For this review, take the finished solid that the model builds, in its own axes (mm). Face numbers are marked on the shaded views. A direction names the side the tool comes from. Give positions to 0.01 mm unless a question says otherwise; leave off trailing zeros. Order: outer loops, then holes, each group sorted by start corner. A loop starts at its lowest first (then second) coordinate and runs counter-clockwise, first axis right, second up.
Autodesk Inventor part; units mm, degrees
ref_plane "YZ Plane" through (0, 0, 0) normal (1, 0, 0) x (0, 1, 0)
ref_plane "XZ Plane" through (0, 0, 0) normal (0, 1, 0) x (-1, 0, 0)
ref_plane "XY Plane" through (0, 0, 0) normal (0, 0, 1) x (1, 0, 0)
sketch "スケッチ3" plane through (0, 0, 0) normal (0, 1, 0) x (-1, 0, 0)
  circle A0 centre (0, 0) radius 3.85
  line L0 (11, -4) -> (4.4721, -4)
  line L1 (-11, -4) -> (-11, -6)
  line L2 (-11, -6) -> (11, -6)
  line L3 (11, -6) -> (11, -4)
  arc A1 (4.4721, -4) -> (-4.4721, -4) centre (0, 0) ccw
  line L4 (-4.4721, -4) -> (-11, -4)
  point P0 (0, -4)
  point P1 (0, -6)
  dimension "d12" = 7.7
  dimension "d14" = 22
  dimension "d15" = 2
  dimension "d16" = 6
extrude "押し出し3" add sketch "スケッチ3" along normal blind 10
sketch "スケッチ4" plane through (4.4721, 0, -4) normal (0, 0, 1) x (1, 0, 0)
  circle A0 centre (4.0279, 7.5) radius 1.05
  circle A1 centre (-12.9721, 2.5) radius 1.05
  line L0 (-15.4721, 0) -> (-15.4721, 10)
  line L1 (6.5279, 0) -> (6.5279, 10)
  line L2 (0, 10) -> (6.5279, 10)
  line L3 (-15.4721, 0) -> (-8.9443, 0)
  line L4 (0, 0) -> (0, 10)
  line L5 (0, 0) -> (6.5279, 0)
  line L6 (0, 0) -> (6.5279, 0)
  line L7 (6.5279, 0) -> (6.5279, 10)
  line L8 (0, 10) -> (6.5279, 10)
  line L9 (0, 0) -> (0, 10)
  line L10 (6.5279, 5) -> (0, 5)
  line L11 (0, 0) -> (6.5279, 0)
  line L12 (6.5279, 5) -> (6.5279, 0)
  line L13 (6.5279, 0) -> (0, 0)
  line L14 (1.5279, 0) -> (-10.4721, 0)
  line L15 (0, 0) -> (0, 5)
  line L16 (-15.4721, 0) -> (-8.9443, 0)
  line L17 (-8.9443, 0) -> (-8.9443, 10)
  line L18 (-15.4721, 10) -> (-8.9443, 10)
  line L19 (-15.4721, 0) -> (-15.4721, 10)
  line L20 (-15.4721, 0) -> (-15.4721, 10)
  line L21 (-15.4721, 10) -> (-8.9443, 10)
  line L22 (-15.4721, 5) -> (-8.9443, 5)
  line L23 (-8.9443, 5) -> (-8.9443, 10)
  line L24 (-8.9443, 10) -> (-15.4721, 10)
  line L25 (-15.4721, 10) -> (-15.4721, 5)
  point P0 (-4.4721, 0)
  dimension "d19" = 2.1
  dimension "d20" = 2.1
  dimension "d21" = 2.5
  dimension "d22" = 2.5
  dimension "d29" = 2.5
  dimension "d30" = 2.5
  dimension "d35" = 17
extrude "押し出し4" cut sketch "スケッチ4" against normal blind 10 contours A0 | A1
sketch "スケッチ5" plane through (0, 10, 0) normal (0, 1, 0) x (1, 0, 0)
  line L0 (-1.5, 0) -> (1.5, 0)
  line L1 (1.5, 0) -> (1.5, 10)
  line L2 (1.5, 10) -> (-1.5, 10)
  line L3 (-1.5, 10) -> (-1.5, 0)
  point P0 (0, 0)
  point P1 (0, 0)
  dimension "d25" = 3
  dimension "d26" = 10
extrude "押し出し5" cut sketch "スケッチ5" against normal blind 10
extrude "押し出し6" cut sketch "スケッチ4" against normal blind 2 contours L4 L10 L1 L5
extrude "押し出し7" cut sketch "スケッチ4" against normal blind 2 contours L0 L18 L17 L22
properties part number "Ω型"
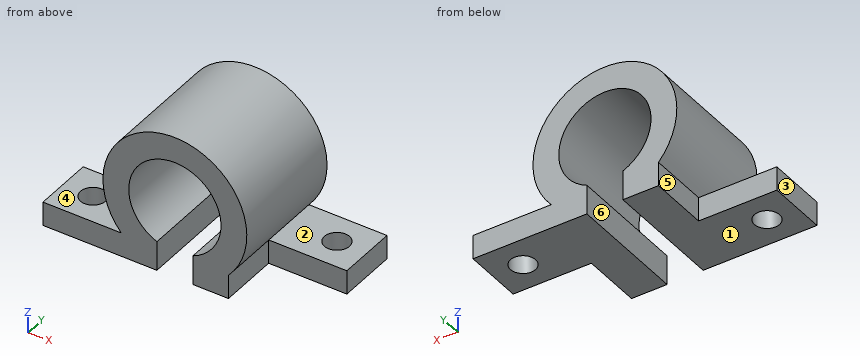
1) Tool access review of the marked faces 4, 5 and 6: name each direction out of +Z, -Z, +X, -X, +Y, -Y from which nothing blocks a thin tool from reaching the whole face with its end or side.
Answer sheet:
face 4: -X, +Y, -Y
face 5: -Z, -X, +Y
face 6: -Z, +Y, -Y
2) We need section A-A on x = 8.5. Give the boundary of the cut face in (y, z).
Answer sheet:
outline: (5, -6) - (6.45, -6) - (6.45, -4) - (5, -4) - close; (8.55, -6) - (10, -6) - (10, -4) - (8.55, -4) - close
3) We need section D-D on y = 4.75. Give the boundary of the cut face in (x, z).
Answer sheet:
outline: (-11, -6) - (-1.5, -6) - (-1.5, -3.55) arc R3.85 cw (long way) to (1.5, -3.55) - (1.5, -6) - (4.47, -6) - (4.47, -4) arc R6 ccw (long way) to (-4.47, -4) - (-11, -4) - close
4) Draft analysis for pull direction Z (two halves, no side actions). For the marked faces 1, 2 and 3, state which applies: +Z half, -Z half, draft (parallel to the pull), parting line (faces both ways), or undercut.
Answer sheet:
face 1: -Z half
face 2: undercut
face 3: draft
5) Clearance check with flat-ended pins moving along their axes: pin 1 (1.5 mm diameter, centred on x = 7.5, y = 8, fed in from +Z); pin 2 (1.2 mm diameter, centred on y = 3.5, z = -5, fed in from +X); pin 3 (1.5 mm diameter, centred on x = 5, y = 5.5, fed in from +Z). State where each tip first meets the part, or that it passes through.
Answer sheet:
pin 1: stops at z = -4
pin 2: stops at x = 4.47
pin 3: stops at z = 4.24
6) We need section C-C on z = -1.5. Give the boundary of the cut face in (x, y).
Answer sheet:
outline: (-5.81, 0) - (-3.55, 0) - (-3.55, 10) - (-5.81, 10) - close; (3.55, 0) - (5.81, 0) - (5.81, 10) - (3.55, 10) - close
7) To check wall thickness, follow line 1 (Y direction, x = 8.5, z = -5.4); line 2 (X direction, y = 4.5, z = 0); line 3 (Y direction, x = -8.5, z = -5.2). State the ranges of each line that lie inside material, in increasing order.
Answer sheet:
line 1: y = 5 to 6.45, 8.55 to 10
line 2: x = -6 to -3.85, 3.85 to 6
line 3: y = 0 to 1.45, 3.55 to 5
